Build history of the part. All positions in model axes, mm. Give positions to 0.01 mm unless a question says otherwise; leave off trailing zeros. Loops run counter-clockwise (first coordinate to the right, second up) from the corner with the lowest first, then second, coordinate; pieces in that order, holes last. Notation, with made-up numbers: (83.25, 38.5) - (120.25, 38.5) arc R38 cw to (120.25, 76.5) - close; hole circle Ø4 at (0.5, -27). An arc over 180 degrees is marked (long way). Return JSON: item names as keys, results as strings. Group by question number.
1) Slice it at A-A (x = 0). List the corners of the cut face in (y, z).
2) Drill centre lines: probe 1 along X at (y, z) = (4.05, -27.5); probe 2 along Z at (x, y) = (-52.5, 3); probe 3 along Z at (x, y) = (-64, 3.6). Where is each one in solid material? Low to high. Write a range as from..to.
3) Drop flat-ended pins along their axis: pin 1 (2.5 mm diameter, centred on x = -21.36, z = -27.34, fed in from -Y); pin 2 (3 mm diameter, centred on y = 4, z = 53.5, fed in from +X); pin 3 (2 mm diameter, centred on x = -18.5, z = 37, fed in from -Y); pin 4 (1 mm diameter, centred on x = 74, y = 1, fed in from +Z). Give the stop position or say it passes through.
4) Slice it at D-D (x = -89.5). List the corners of the cut face in (y, z).
5) Slice it at C-C (y = 1.8). Count the separate pieces of the cut face and the enclosed holes in it, and give its area (3 significant figures).
6) Slice it at B-B (z = 66). List the corners of the cut face in (x, y).
7) Mould opens along Z. For faces 1 (the face through (22, 0, -1)), 2 (the face through (-1, 2, 94)), 3 (the face through (-7.7, 2.5, -10.1)), 4 (the face through (-81.045, 2.465, -47.626)) say: released by +Z, released by -Z, zero draft, split by the parting line, or undercut.
```python
from build123d import *

# Parameters (mm, degrees)
BOSS_EXTRUDE1_DEPTH = 5
CUT_EXTRUDE3_DEPTH  = 144.674400411
SKETCH7_R           = 1.5
CUT_EXTRUDE5_DEPTH  = 144.674400411
CIRPATTERN3_DEPTH   = 5
CUT_EXTRUDE6_REACH  = 145.04
SKETCH9_R           = 12.7
SKETCH10_R          = 1.5
CUT_EXTRUDE7_DEPTH  = 144.040070255


# Read off the part's stored shape, not the designer's step: CirPattern3
with BuildPart() as part:
    # Sketch1 → Boss-Extrude1 (new body)
    with BuildSketch(Plane(origin=(0, 0, 0), x_dir=(1, 0, 0), z_dir=(0, 1, 0))):
        Polygon((54.270925304, 94), (-54.270925304, 94), (-108.541850608, 0), (-54.270925304, -94), (54.270925304, -94), (108.541850608, 0), align=None)
    extrude(amount=BOSS_EXTRUDE1_DEPTH)

    # Sketch6 → Cut-Extrude3 (cut, through all)
    with BuildSketch(Plane(origin=(0, 5, 0), x_dir=(1, 0, 0), z_dir=(0, 1, 0))):
        Polygon((-52.550395529, 93.006651671), (-52.550395529, 94.993348329), (-54.270925304, 95.986696658), (-55.991455079, 94.993348329), (-55.991455079, 93.006651671), (-54.270925304, 92.013303342), align=None)
    extrude(amount=-CUT_EXTRUDE3_DEPTH, mode=Mode.SUBTRACT)

    # Sketch7 → Cut-Extrude5 (cut, through all)
    with BuildSketch(Plane(origin=(0, 5, 0), x_dir=(1, 0, 0), z_dir=(0, 1, 0))):
        with Locations((-53.4048999, 92.5)):
            Circle(SKETCH7_R)
    extrude(amount=-CUT_EXTRUDE5_DEPTH, mode=Mode.SUBTRACT)

    # CirPattern3 outline → CirPattern3 (cut)
    with BuildSketch(Plane(origin=(0, 0, 0), x_dir=(1, 0, 0), z_dir=(0, 1, 0))):
        with BuildLine():
            ThreePointArc((107.490156817, 1.335134155), (105.331435102, -0.002284917), (107.471793734, -1.368899034))
            Line((107.471793734, -1.368899034), (107.68158572, -1.490022493))
            Line((107.68158572, -1.490022493), (108.541850608, 0))
            Line((108.541850608, 0), (107.700797112, 1.456747386))
            Line((107.700797112, 1.456747386), (107.490156817, 1.335134155))
        make_face()
        with BuildLine():
            Line((54.913619301, 92.369573958), (55.137593989, 92.498885804))
            Line((55.137593989, 92.498885804), (54.270925304, 94))
            Line((54.270925304, 94), (52.576010718, 94))
            Line((52.576010718, 94), (52.576010718, 93.740508989))
            ThreePointArc((52.576010718, 93.740508989), (52.660468715, 91.206101044), (54.913619301, 92.369573958))
        make_face()
        with BuildLine():
            Line((-108.541850608, 0), (-107.675181923, -1.501114196))
            Line((-107.675181923, -1.501114196), (-107.451207235, -1.37180235))
            ThreePointArc((-107.451207235, -1.37180235), (-105.317034842, -0.002253161), (-107.469667507, 1.338093583))
            Line((-107.469667507, 1.338093583), (-107.694393315, 1.467839088))
            Line((-107.694393315, 1.467839088), (-108.541850608, 0))
        make_face()
        with BuildLine():
            Line((-54.270925304, -94), (-52.550395529, -94))
            Line((-52.550395529, -94), (-52.550395529, -93.757753081))
            ThreePointArc((-52.550395529, -93.757753081), (-52.663738755, -91.220841074), (-54.901338504, -92.421639383))
            Line((-54.901338504, -92.421639383), (-55.111978799, -92.543252614))
            Line((-55.111978799, -92.543252614), (-54.270925304, -94))
        make_face()
        with BuildLine():
            Line((54.270925304, -94), (55.118382597, -92.532160912))
            Line((55.118382597, -92.532160912), (54.915257504, -92.414886585))
            ThreePointArc((54.915257504, -92.414886585), (52.669300376, -91.225904252), (52.576010718, -93.765451347))
            Line((52.576010718, -93.765451347), (52.576010718, -94))
            Line((52.576010718, -94), (54.270925304, -94))
        make_face()
    extrude(amount=CIRPATTERN3_DEPTH, mode=Mode.SUBTRACT)

    # Sketch9 → Cut-Extrude6 (cut, up to next)
    with BuildSketch(Plane(origin=(0, 5, 0), x_dir=(1, 0, 0), z_dir=(0, 1, 0)), mode=Mode.PRIVATE) as cut_extrude6_sk1:
        with Locations(Location((0, 0, 0), (0, 0, 270))):
            Circle(SKETCH9_R)
    cut_extrude6_tool1 = extrude(cut_extrude6_sk1.sketch, amount=-CUT_EXTRUDE6_REACH, mode=Mode.PRIVATE) & part.part
    add(cut_extrude6_tool1.solids().sort_by_distance((0, 5, 0))[0], mode=Mode.SUBTRACT)

    # Sketch10 → Cut-Extrude7 (cut, through all)
    with BuildSketch(Plane(origin=(0, 5, 0), x_dir=(1, 0, 0), z_dir=(0, 1, 0))):
        with Locations(Location((-68.463084387, -51.348426962, 0), (0, 0, 270))):
            Circle(SKETCH10_R)
        with Locations(Location((-10.2375, 84.964983782, 0), (0, 0, 270))):
            Circle(SKETCH10_R)
        with Locations(Location((-21.3625, 27.339983782, 0), (0, 0, 270))):
            Circle(SKETCH10_R)
        with Locations(Location((-10.2375, 27.339983782, 0), (0, 0, 270))):
            Circle(SKETCH10_R)
        with Locations(Location((-21.3625, 84.964983782, 0), (0, 0, 270))):
            Circle(SKETCH10_R)
        with Locations(Location((28.795870494, -4.80405682, 0), (0, 0, 270))):
            Circle(SKETCH10_R)
        with Locations(Location((34.358370494, 4.830475797, 0), (0, 0, 270))):
            Circle(SKETCH10_R)
        with Locations(Location((84.263084387, -23.982024203, 0), (0, 0, 270))):
            Circle(SKETCH10_R)
        with Locations(Location((78.700584387, -33.61655682, 0), (0, 0, 270))):
            Circle(SKETCH10_R)
        with Locations(Location((-12.995870494, -32.170459579, 0), (0, 0, 270))):
            Circle(SKETCH10_R)
        with Locations(Location((-18.558370494, -22.535926962, 0), (0, 0, 270))):
            Circle(SKETCH10_R)
        with Locations(Location((-62.900584387, -60.982959579, 0), (0, 0, 270))):
            Circle(SKETCH10_R)
    extrude(amount=-CUT_EXTRUDE7_DEPTH, mode=Mode.SUBTRACT)


solid = part.part
```
Results:
{
 "1": {"outline": "(0, -94) - (5, -94) - (5, -12.7) - (0, -12.7) - close; (0, 12.7) - (5, 12.7) - (5, 94) - (0, 94) - close"},
 "2": {"probe 1": "-92.66..-22.85, -19.87..-11.73, -8.75..92.66", "probe 2": "-94..-93.7, -91.3..91.33, 93.72..94", "probe 3": "-77.15..59.96, 62..77.15"},
 "3": {"pin 1": "through", "pin 2": "x = 78.52", "pin 3": "y = 0", "pin 4": "z = 60.69"},
 "4": {"outline": "(0, -32.98) - (5, -32.98) - (5, 32.98) - (0, 32.98) - close"},
 "5": {"separate pieces": "1", "enclosed holes": "13", "area": "30,000 mm2"},
 "6": {"outline": "(-70.44, 0) - (70.44, 0) - (70.44, 5) - (-70.44, 5) - close"},
 "7": {"face 1": "zero draft", "face 2": "released by +Z", "face 3": "undercut", "face 4": "released by -Z"}
}
